```python
from build123d import *

# Parameters (mm, degrees)
F0_R           = 3.175
F1_DEPTH       = 88.9
F4_D           = 2.7051
F4_DEPTH       = 15.08125
F4_TIP         = 0.8126940303
F4_ON_F2_D     = 2.7051
F4_ON_F2_DEPTH = 15.08125
F4_ON_F2_TIP   = 0.8126940303


with BuildPart() as f1:
    # F0 (on Front) → F1 (new body)
    with BuildSketch(Plane.XZ):
        Circle(F0_R)
    extrude(amount=F1_DEPTH)

    # F4
    with Locations(Plane(origin=(0, 0, 0), x_dir=(-1, 0, 0), z_dir=(0, 1, 0))):
        with Locations((0, 0)):
            Hole(F4_D / 2, depth=F4_DEPTH)
            with Locations((0, 0, -(F4_DEPTH + F4_TIP / 2))):  # 118° drill point
                Cone(0, F4_D / 2, F4_TIP, mode=Mode.SUBTRACT)

    # F4 on F2
    with Locations(Plane.XZ.offset(88.9)):
        with Locations((0, 0)):
            Hole(F4_ON_F2_D / 2, depth=F4_ON_F2_DEPTH)
            with Locations((0, 0, -(F4_ON_F2_DEPTH + F4_ON_F2_TIP / 2))):  # 118° drill point
                Cone(0, F4_ON_F2_D / 2, F4_ON_F2_TIP, mode=Mode.SUBTRACT)


solid = f1.part
```
Could you check a few things on this model? Use its own coordinates, in mm. A direction names the side the tool comes from. Round coordinates to 2 decimals unless told otherwise and drop trailing zeros. Loops run counter-clockwise (first coordinate to the right, second up) from the corner with the lowest first, then second, coordinate; pieces in that order, holes last. Notation, with made-up numbers: M -26,82 L 12,82 A25 cw 12,112 Z; hole C 72.5,32 d1. An arc over 180 degrees is marked long. Write item = value, one per line.
1. I want a section at B-B, the plane z = -2.25. Write out the boundary of the cut face in (x, y).
Results below:
outline = M -2.24,-88.9 L 2.24,-88.9 L 2.24,0 L -2.24,0 Z
2. I need wall thicknesses on probe 1 along Z at (x, y) = (0, -6.5) (3 decimals); probe 2 along X at (y, z) = (-25.5, -0.25); probe 3 along Z at (x, y) = (0.75, -80). Which ranges of each line are inside material? Lowest first, please.
Results below:
probe_1 = -3.175 to -1.353, 1.353 to 3.175
probe_2 = -3.17 to 3.17
probe_3 = -3.09 to -1.13, 1.13 to 3.09
3. Which directions (+Z, -Z, +X, -X, +Y, -Y) give clear straight access to the entire face, cutting with the end or side of a thin tool? Please do faces 5 (the face through (1.4, 0, -0.7)), 6 (the face through (-1.29, -81.25, 0.41)).
Results below:
face_5 = +Z, -Z, +X, -X, +Y
face_6 = -Y
4. Will this pin go through, and if not, where does the flat tip stop? P1, Ø1.6, axis at x = 0, z = 0, coming from the +Y side.
Results below:
P1 = -15.41
5. I want a section at A-A, the plane y = -42. Write out the boundary of the cut face in (x, z) (3 decimals), and give its area (3 significant figures).
Results below:
outline = C 0,0 d6.35
area = 31.7 mm²
6. Thinking about a two-plate mould opening in X: for faces 1 (the face through (1.4, -88.9, -0.7)), 2 (the face through (1.29, -7.65, 0.41)), 3 (the face through (-0.69, -43.83, -3.1)), 4 (the face through (-0.224, -15.753, 0.071)), which applies, +X half, -X half, draft (parallel to the pull), parting line (faces both ways), or undercut?
Results below:
face_1 = draft
face_2 = undercut
face_3 = parting line
face_4 = undercut
